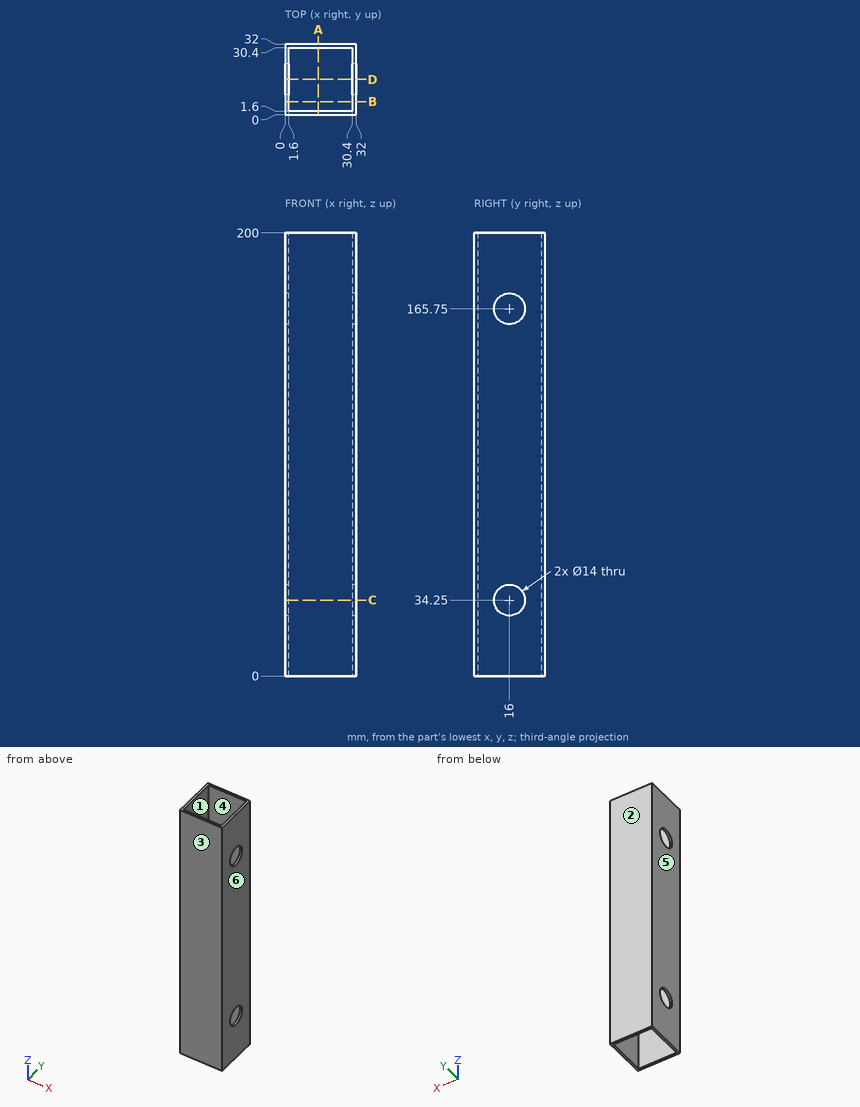
Answer from the drawing. Dimensions are ordinates in mm from the lowest x, y and z of the part. A direction names the side the tool comes from. Coordinates: 2 decimals unless noted, no trailing zeros. Write each loop counter-clockwise with the first axis right and the second up, starting at its lowest first coordinate (ties: lowest second). Pieces come first, ordered by that corner, then holes. Notation, with made-up numbers: M 17,5.25 L 41,5.25 A18 ccw 41,29.25 Z; hole C 77,28.25 d6. An arc over 180 degrees is marked long. Put each result on its own line as item: value. Start each with the question number.
1. A cutting plane is placed at C-C on z = 34.25. Write down the section's boundary in (x, y), then the cut area to 3 significant figures.
2. For a pull along X with two mould halves and no side action, classify the marked faces 3, 4, 5 and 6 as pulls with the +X half, pulls with the -X half, needs draft (parallel to the pull), parting line crosses it, or undercut.
3. Which of the six approach directions +Z, -Z, +X, -X, +Y, -Y give full straight-line access (tool end or side, diameter ignored) to the marked faces 1 and 2?
4. Consider line 1 (Z direction, x = 0.9, y = 16); line 2 (X direction, y = 2.5, z = 20). Determine where each line is inside the solid, lowest interval first. Write a range as from..to.
5. A cutting plane is placed at D-D on y = 16. Write down the section's boundary in (x, z), then the cut area to 3 significant figures.
6. A cutting plane is placed at A-A on x = 15. Write down the section's boundary in (y, z).
Resolved:
1. outline: M 0,0 L 32,0 L 32,9 L 30.4,9 L 30.4,1.6 L 1.6,1.6 L 1.6,9 L 0,9 Z; M 0,23 L 1.6,23 L 1.6,30.4 L 30.4,30.4 L 30.4,23 L 32,23 L 32,32 L 0,32 Z
1. area: 150 mm2
2. face 3: needs draft
2. face 4: undercut
2. face 5: pulls with the -X half
2. face 6: pulls with the +X half
3. face 1: +Z, -Z
3. face 2: +Z, -Z, +X, -X, +Y
4. line 1: z = 0..27.25, 41.25..158.75, 172.75..200
4. line 2: x = 0..1.6, 30.4..32
5. outline: M 0,0 L 1.6,0 L 1.6,27.25 L 0,27.25 Z; M 0,41.25 L 1.6,41.25 L 1.6,158.75 L 0,158.75 Z; M 0,172.75 L 1.6,172.75 L 1.6,200 L 0,200 Z; M 30.4,0 L 32,0 L 32,27.25 L 30.4,27.25 Z; M 30.4,41.25 L 32,41.25 L 32,158.75 L 30.4,158.75 Z; M 30.4,172.75 L 32,172.75 L 32,200 L 30.4,200 Z
5. area: 550 mm2
6. outline: M 0,0 L 1.6,0 L 1.6,200 L 0,200 Z; M 30.4,0 L 32,0 L 32,200 L 30.4,200 Z
